CAD build for the part. Positions are in the model's coordinates, mm. Face numbers are marked on the shaded views. A direction names the side the tool comes from. Give positions to 0.01 mm unless a question says otherwise; leave off trailing zeros. Write each loop counter-clockwise with the first axis right and the second up, starting at its lowest first coordinate (ties: lowest second). Pieces come first, ordered by that corner, then holes. Notation, with made-up numbers: (17.5, -8) -> (33.5, -8) arc R25 cw to (33.5, 26) -> close; hole circle Ø3 at (-37, 6.5). An arc over 180 degrees is marked (long way). Answer as a JSON object with one key per item and string values.
```python
from build123d import *

# Parameters (mm, degrees)
F0_R     = 47
F0_R_2   = 2.5
F0_R_3   = 25
F1_DEPTH = 5
F2_R     = 35
F2_R_2   = 25
F3_DEPTH = 2
F4_R     = 46
F5_DEPTH = 1


with BuildPart() as f1:
    # F0 (on Top) → F1 (new body)
    with BuildSketch(Plane.XY):
        Circle(F0_R)
        with Locations((-35.940054, -20.75)):
            Circle(F0_R_2, mode=Mode.SUBTRACT)
        with Locations((0, -41.5)):
            Circle(F0_R_2, mode=Mode.SUBTRACT)
        with Locations((35.940054, -20.75)):
            Circle(F0_R_2, mode=Mode.SUBTRACT)
        with Locations((-35.940054, 20.75)):
            Circle(F0_R_2, mode=Mode.SUBTRACT)
        Circle(F0_R_3, mode=Mode.SUBTRACT)
        with Locations((35.940054, 20.75)):
            Circle(F0_R_2, mode=Mode.SUBTRACT)
        with Locations((0, 41.5)):
            Circle(F0_R_2, mode=Mode.SUBTRACT)
    extrude(amount=F1_DEPTH)

    # F2 (on face) → F3 (join)
    with BuildSketch(Plane.XY.offset(5)):
        Circle(F2_R)
        Circle(F2_R_2, mode=Mode.SUBTRACT)
    extrude(amount=F3_DEPTH)

    # F4 (on face) → F5 (cut)
    with BuildSketch(Plane(origin=(0, 0, 0), x_dir=(1, 0, 0), z_dir=(0, 0, -1))):
        Circle(F4_R)
    extrude(amount=-F5_DEPTH, mode=Mode.SUBTRACT)


solid = f1.part
```
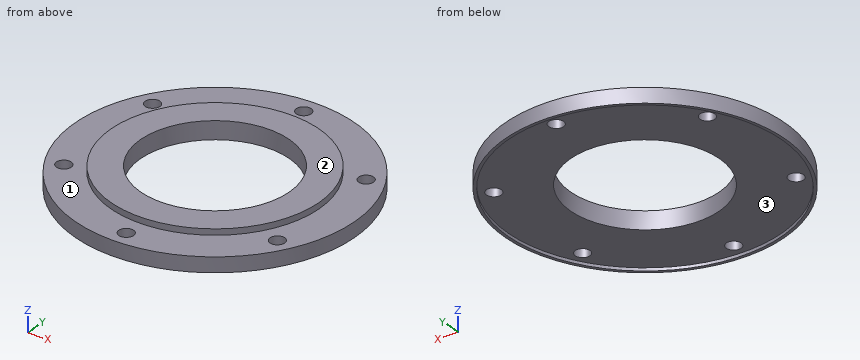
1) Slice it at A-A (y = 0). List the corners of the cut face in (x, z).
Model answer:
{"outline": "(-47, 0) -> (-46, 0) -> (-46, 1) -> (-25, 1) -> (-25, 7) -> (-35, 7) -> (-35, 5) -> (-47, 5) -> close; (25, 1) -> (46, 1) -> (46, 0) -> (47, 0) -> (47, 5) -> (35, 5) -> (35, 7) -> (25, 7) -> close"}
2) 3-axis set-ups, long thin cutter, end or side, ignore diameter. For the marked faces 1, 2 and 3: which of +Z, -Z, +X, -X, +Y, -Y reach the whole face in a straight line?
Model answer:
{"face 1": "+Z", "face 2": "+Z, +X, -X, +Y, -Y", "face 3": "-Z"}
3) Slice it at B-B (x = 0). List the corners of the cut face in (y, z).
Model answer:
{"outline": "(-47, 0) -> (-46, 0) -> (-46, 1) -> (-44, 1) -> (-44, 5) -> (-47, 5) -> close; (-39, 1) -> (-25, 1) -> (-25, 7) -> (-35, 7) -> (-35, 5) -> (-39, 5) -> close; (25, 1) -> (39, 1) -> (39, 5) -> (35, 5) -> (35, 7) -> (25, 7) -> close; (44, 1) -> (46, 1) -> (46, 0) -> (47, 0) -> (47, 5) -> (44, 5) -> close"}
4) Wall check: probe 1 along Y at (x, z) = (0, 4.55); probe 2 along Y at (x, z) = (0, 0.35); probe 3 along X at (y, z) = (-20.75, 3). Give the ranges that are in metal, low to high.
Model answer:
{"probe 1": "y = -47 to -44, -39 to -25, 25 to 39, 44 to 47", "probe 2": "y = -47 to -46, 46 to 47", "probe 3": "x = -42.17 to -38.44, -33.44 to -13.94, 13.94 to 33.44, 38.44 to 42.17"}
5) Pin check, flat tips, straight feed: pin 1 (1.5 mm diameter, centred on x = 16, y = 25.5, fed in from -Z); pin 2 (3 mm diameter, centred on x = 35.94, y = -20.75, fed in from -Z); pin 3 (2 mm diameter, centred on x = -14.5, z = 3.5, fed in from +Y); pin 4 (1.5 mm diameter, centred on x = 21.5, z = 6, fed in from -Y). Stop position of each tip, or through.
Model answer:
{"pin 1": "stops at z = 1", "pin 2": "passes through", "pin 3": "stops at y = 45.02", "pin 4": "stops at y = -28.19"}
6) Slice it at C-C (z = 2.5). List the corners of the cut face in (x, y).
Model answer:
{"outline": "circle Ø94 at (0, 0); hole circle Ø5 at (-35.94, -20.75); hole circle Ø5 at (-35.94, 20.75); hole circle Ø50 at (0, 0); hole circle Ø5 at (0, -41.5); hole circle Ø5 at (0, 41.5); hole circle Ø5 at (35.94, -20.75); hole circle Ø5 at (35.94, 20.75)"}
7) Slice it at D-D (x = -10). List the corners of the cut face in (y, z), then the cut area to 3 significant figures.
Model answer:
{"outline": "(-45.92, 0) -> (-44.9, 0) -> (-44.9, 1) -> (-22.91, 1) -> (-22.91, 7) -> (-33.54, 7) -> (-33.54, 5) -> (-45.92, 5) -> close; (22.91, 1) -> (44.9, 1) -> (44.9, 0) -> (45.92, 0) -> (45.92, 5) -> (33.54, 5) -> (33.54, 7) -> (22.91, 7) -> close", "area": "229 mm2"}
